Geometry: final body of the model. Coordinates: model frame, mm. Face numbers are marked on the shaded views. A direction names the side the tool comes from. Round coordinates to 2 decimals unless told otherwise and drop trailing zeros. Loops run counter-clockwise (first coordinate to the right, second up) from the corner with the lowest first, then second, coordinate; pieces in that order, holes last. Notation, with made-up numbers: (5.25, -7) -> (52.25, -7) arc R29 ccw to (52.25, 30) -> close; hole circle Ø5 at (32.25, -40). An arc over 180 degrees is marked (long way). Answer in a Markdown table with one row per item.
```python
from build123d import *

# Parameters (mm, degrees)
SKETCH2_W           = 32
SKETCH2_H           = 12
BOSS_EXTRUDE1_DEPTH = 3
SKETCH3_W           = 7
SKETCH3_H           = 3
SKETCH3_W_2         = 3
SKETCH3_H_2         = 6
BOSS_EXTRUDE3_DEPTH = 3
SKETCH4_W           = 2.2
SKETCH4_H           = 8
CUT_EXTRUDE1_DEPTH  = 3


with BuildPart() as part:
    # Sketch2 → Boss-Extrude1 (new body)
    with BuildSketch(Plane.XY):
        Rectangle(SKETCH2_W, SKETCH2_H)
    extrude(amount=BOSS_EXTRUDE1_DEPTH)

    # Sketch3 → Boss-Extrude3 (add)
    with BuildSketch(Plane.XY.offset(3)):
        with Locations((-6.5, -7.5)):
            Rectangle(SKETCH3_W, SKETCH3_H)
        with Locations((6.5, -7.5)):
            Rectangle(SKETCH3_W, SKETCH3_H)
        with Locations((6.5, 7.5)):
            Rectangle(SKETCH3_W, SKETCH3_H)
        with Locations((-6.5, 7.5)):
            Rectangle(SKETCH3_W, SKETCH3_H)
        with Locations((-17.5, 0)):
            Rectangle(SKETCH3_W_2, SKETCH3_H_2)
        with Locations((17.5, 0)):
            Rectangle(SKETCH3_W_2, SKETCH3_H_2)
    extrude(amount=-BOSS_EXTRUDE3_DEPTH)

    # Sketch4 → Cut-Extrude1 (cut)
    with BuildSketch(Plane.XY.offset(3)):
        with Locations((-13.35, 0)):
            Rectangle(SKETCH4_W, SKETCH4_H)
    extrude(amount=-CUT_EXTRUDE1_DEPTH, mode=Mode.SUBTRACT)


solid = part.part
```
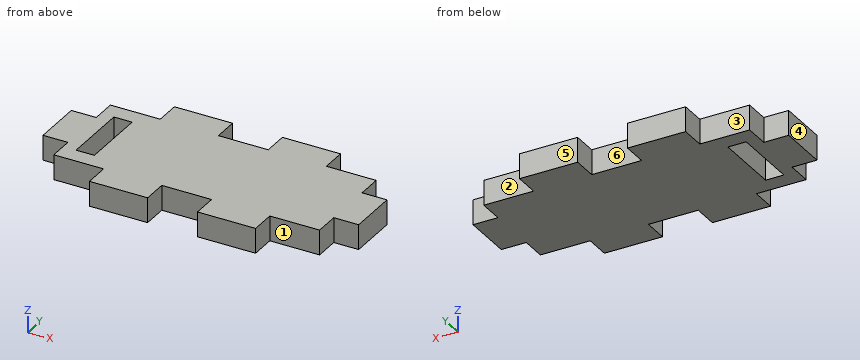
Item 1: Section query D-D, the plane x = 15. Output: boundary loops of the cut face in (y, z).
Ans:
| item | result |
|---|---|
| outline | (-6, 0) -> (6, 0) -> (6, 3) -> (-6, 3) -> close |
Item 2: Ray query, L1, parallel to X at y = -0.5, z = 0.85; L2, parallel to X at y = -7, z = 0.9; L3, parallel to Y at x = -13, z = 0.55. Return the intervals inside material, ascending.
Ans:
| item | result |
|---|---|
| L1 | -19 to -14.45, -12.25 to 19 |
| L2 | -10 to -3, 3 to 10 |
| L3 | -6 to -4, 4 to 6 |
Item 3: Mould query, pull axis X, two halves, no side actions, for the marked faces 4, 5 and 6. Classes: released by +X, released by -X, zero draft, split by the parting line, or undercut.
Ans:
| item | result |
|---|---|
| face 4 | released by -X |
| face 5 | zero draft |
| face 6 | undercut |
Item 4: Set-up query: the marked faces 1, 2 and 3. Return all of +Z, -Z, +X, -X, +Y, -Y with unobstructed straight access to the full face (end or side cutting, diameter ignored); none if empty.
Ans:
| item | result |
|---|---|
| face 1 | +Z, -Z, +X, -Y |
| face 2 | +Z, -Z, +X, +Y |
| face 3 | +Z, -Z, -X, +Y |
Item 5: First-contact query: P1, Ø4, axis at x = -7, y = -6, coming from the -Z side; P2, Ø1.5, axis at x = 0.5, z = 1, coming from the +Y side; P3, Ø0.9, axis at y = -7, z = 1.5, coming from the +X side; P4, Ø1.5, axis at y = 4.5, z = 1.5, coming from the -X side. Flat tips, straight axial feed; report the tip coordinate or a pass-through.
Ans:
| item | result |
|---|---|
| P1 | z = 0 |
| P2 | y = 6 |
| P3 | x = 10 |
| P4 | x = -16 |
Item 6: Section query A-A, the plane y = 6.5. Output: boundary loops of the cut face in (x, z).
Ans:
| item | result |
|---|---|
| outline | (-10, 0) -> (-3, 0) -> (-3, 3) -> (-10, 3) -> close; (3, 0) -> (10, 0) -> (10, 3) -> (3, 3) -> close |
Item 7: Section query C-C, the plane y = 0. Output: boundary loops of the cut face in (x, z).
Ans:
| item | result |
|---|---|
| outline | (-19, 0) -> (-14.45, 0) -> (-14.45, 3) -> (-19, 3) -> close; (-12.25, 0) -> (19, 0) -> (19, 3) -> (-12.25, 3) -> close |
